The drawing under review shows one solid part. Ordinate dimensions are in mm from its lowest x, y, z. Round coordinates to 2 decimals unless told otherwise and drop trailing zeros. Loops run counter-clockwise (first coordinate to the right, second up) from the corner with the lowest first, then second, coordinate; pieces in that order, holes last. Notation, with made-up numbers: (47, 20.5) -> (81, 20.5) arc R24 cw to (81, 43.5) -> close; hole circle Ø10 at (-16, 7.5). An arc over 180 degrees is marked (long way). Answer as CSV lines item,"result". Start each with the question number.
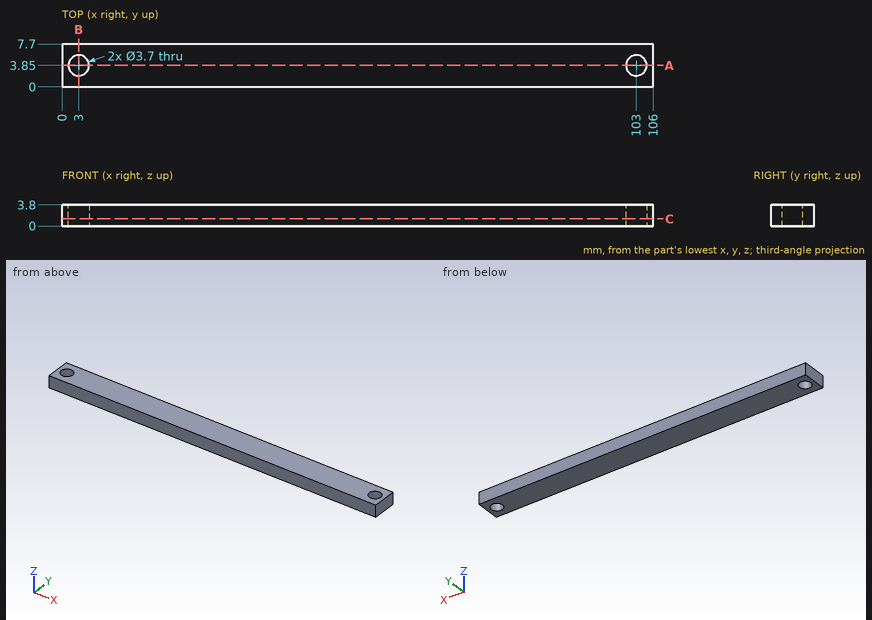
Q1. To check wall thickness, follow probe 1 along X at (y, z) = (3.75, 3.1); probe 2 along Y at (x, z) = (3, 1.7); probe 3 along X at (y, z) = (5, 1.35). State the ranges of each line that lie inside material, in increasing order. Write a range as from..to.
Q2. Add section C-C, the plane z = 1.3. Give the boundary of the cut face in (x, y).
Q3. Add section A-A, the plane y = 3.85. Give the boundary of the cut face in (x, z), and give its area (3 significant figures).
Q4. Add section B-B, the plane x = 3. Give the boundary of the cut face in (y, z), and give its area (3 significant figures).
Q5. For pin 1 Ø3.5 at (x, y) = (3, 3.85) entering from +Z, flat-tipped, find the tip position at first contact; note if it passes through.
Worked answers:
1,probe 1,"x = 0..1.15, 4.85..101.15, 104.85..106"
1,probe 2,"y = 0..2, 5.7..7.7"
1,probe 3,"x = 0..1.55, 4.45..101.55, 104.45..106"
2,outline,"(0, 0) -> (106, 0) -> (106, 7.7) -> (0, 7.7) -> close; hole circle Ø3.7 at (3, 3.85); hole circle Ø3.7 at (103, 3.85)"
3,outline,"(0, 0) -> (1.15, 0) -> (1.15, 3.8) -> (0, 3.8) -> close; (4.85, 0) -> (101.15, 0) -> (101.15, 3.8) -> (4.85, 3.8) -> close; (104.85, 0) -> (106, 0) -> (106, 3.8) -> (104.85, 3.8) -> close"
3,area,"375 mm^2"
4,outline,"(0, 0) -> (2, 0) -> (2, 3.8) -> (0, 3.8) -> close; (5.7, 0) -> (7.7, 0) -> (7.7, 3.8) -> (5.7, 3.8) -> close"
4,area,"15.2 mm^2"
5,pin 1,"passes through"
